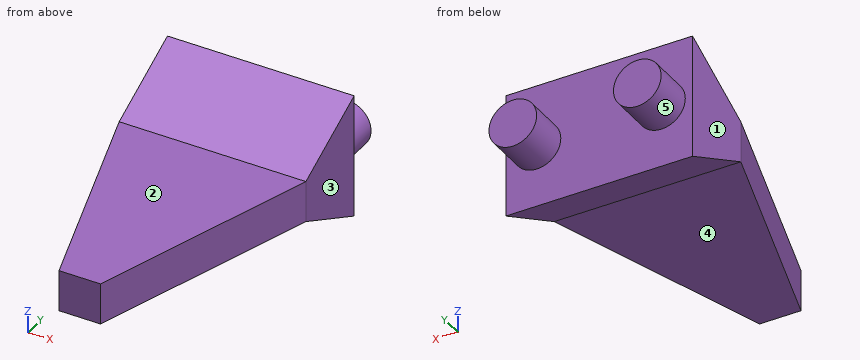
```python
from build123d import *

# Parameters (mm, degrees)
F0_W          = 9
F0_H          = 4
F1_DEPTH      = 2
F2_DEPTH      = 4
F2_DEPTH_BACK = 2
F3_SIZE2      = 3.99999
F3_SIZE       = 1.99999
F4_SIZE2      = 3.99999
F4_SIZE       = 1.99999
F5_R          = 1.15
F6_DEPTH      = 2


# Not quite as in the source:
# - a fillet or chamfer is up to 0.001 mm smaller than in the source, because OpenCascade refuses the exact size


with BuildPart() as f1:
    # F0 (on Top) → F1 (new body)
    with BuildSketch(Plane.XY):
        with Locations((0, 5.5)):
            Rectangle(F0_W, F0_H)
        Polygon((1, -7.5), (4.5, 3.5), (-4.5, 3.5), (-1, -7.5), align=None)
    extrude(amount=F1_DEPTH)

    # F0 (on Top) → F2 (join, two sides)
    with BuildSketch(Plane.XY) as f2_sk:
        with Locations((0, 5.5)):
            Rectangle(F0_W, F0_H)
    extrude(amount=F2_DEPTH)
    extrude(f2_sk.sketch, amount=-F2_DEPTH_BACK)

    # F3 (size 2 and 4 in the source; OpenCascade refuses exactly that, so slightly less here)
    f3_edges = [f1.edges().sort_by_distance(p)[0] for p in [
        (0, 3.5, -2),
    ]]
    f3_side = f1.faces().sort_by_distance((0, 3.5, -1))[0]
    chamfer(f3_edges, length=F3_SIZE, length2=F3_SIZE2, reference=f3_side)

    # F4 (size 2 and 4 in the source; OpenCascade refuses exactly that, so slightly less here)
    f4_edges = [f1.edges().sort_by_distance(p)[0] for p in [
        (0, 3.5, 4),
    ]]
    f4_side = f1.faces().sort_by_distance((0, 3.5, 3))[0]
    chamfer(f4_edges, length=F4_SIZE, length2=F4_SIZE2, reference=f4_side)

    # F5 (on face) → F6 (join)
    with BuildSketch(Plane(origin=(0, 7.5, 0), x_dir=(-1, 0, 0), z_dir=(0, 1, 0))):
        with Locations((-3, 1)):
            Circle(F5_R)
        with Locations((3, 1)):
            Circle(F5_R)
    extrude(amount=F6_DEPTH)


solid = f1.part
```
Design review of the part built by this model. Coordinates are the model's own, in mm. Face numbers are marked on the shaded views. A direction names the side the tool comes from. Coordinates: 2 decimals unless noted, no trailing zeros. Order: outer loops, then holes, each group sorted by start corner. A loop starts at its lowest first (then second) coordinate and runs counter-clockwise, first axis right, second up. Notation, with made-up numbers: (55, 20) - (89, 20) arc R26 ccw to (89, 47) - close; hole circle Ø9 at (-17.75, 71). An arc over 180 degrees is marked (long way). One line per question, with ' | ' between items.
Q1. Consider section D-D, the plane y = 7. Give the boundary of the cut face in (x, z), then the cut area to 3 significant figures.
Answer key:
outline: (-4.5, -1.75) - (4.5, -1.75) - (4.5, 3.75) - (-4.5, 3.75) - close | area: 49.5 mm2
Q2. Consider section C-C, the plane y = 4.5. Give the boundary of the cut face in (x, z).
Answer key:
outline: (-4.5, -0.5) - (4.5, -0.5) - (4.5, 2.5) - (-4.5, 2.5) - close
Q3. Consider section A-A, the plane z = 1. Give the boundary of the cut face in (x, y), then the cut area to 3 significant figures.
Answer key:
outline: (-4.5, 3.5) - (-1, -7.5) - (1, -7.5) - (4.5, 3.5) - (4.5, 7.5) - (4.15, 7.5) - (4.15, 9.5) - (1.85, 9.5) - (1.85, 7.5) - (-1.85, 7.5) - (-1.85, 9.5) - (-4.15, 9.5) - (-4.15, 7.5) - (-4.5, 7.5) - close | area: 106 mm2
Q4. Clearance check with flat-ended pins moving along their axes: pin 1 Ø4.5 at (x, y) = (0.5, -1.5) entering from +Z; pin 2 Ø3 at (x, z) = (1.5, 0.5) entering from +Y. State where each tip first meets the part, or that it passes through.
Answer key:
pin 1: stops at z = 2 | pin 2: stops at y = 9.5
Q5. For the marked faces 1, 2, 3, 4 and 5, list the 3-axis set-ups (+Z, -Z, +X, -X, +Y, -Y) from which the entire face can be reached by the end or side of a thin tool; tool diameter is ignored.
Answer key:
face 1: +Z, -Z, -X, +Y, -Y | face 2: +Z, +X, -X, -Y | face 3: +Z, -Z, +X, +Y, -Y | face 4: -Z, +X, -X, -Y | face 5: +Y
Q6. To check wall thickness, follow line 1 along Z through (x, y) = (0, -5); line 2 along Y through (x, z) = (3.25, 2.5); line 3 along X through (y, z) = (-3, 1.75). State the ranges of each line that lie inside material, in increasing order.
Answer key:
line 1: z = 0 to 2 | line 2: y = 4.5 to 7.5 | line 3: x = -2.43 to 2.43
